Here's how the part is built. I have some questions about the finished solid (model axes, mm). Face numbers are marked on the shaded views. A direction names the side the tool comes from. Round coordinates to 2 decimals unless told otherwise and drop trailing zeros. Loops run counter-clockwise (first coordinate to the right, second up) from the corner with the lowest first, then second, coordinate; pieces in that order, holes last. Notation, with made-up numbers: (70.5, -0.75) - (95.5, -0.75) arc R32 cw to (95.5, 35.25) - close; hole circle Ø8 at (3.25, 58.25). An arc over 180 degrees is marked (long way). Answer as a JSON object with one key per item and string values. Group by question number.
1) If we mould it in two halves opening along Y, with no side actions, what happens to the marked faces 4, 5 and 6? For each: pulls with the +Y half, pulls with the -Y half, needs draft (parallel to the pull), parting line crosses it, or undercut.
2) I want a section at B-B, the plane y = -7.5. Please give me the cut outline in (x, z) (3 decimals), then the cut area to 3 significant figures.
3) If I drill on line 1 along Y through (x, z) = (19.05, 30.75); line 2 along Z through (x, y) = (17.5, 28); line 3 along Y through (x, z) = (23, 17.5), over which ranges is the centre line in solid material (lowest first)? Write a range as [from, to].
4) I want a section at D-D, the plane z = 21. Please give me the cut outline in (x, y), then the cut area to 3 significant figures.
5) I want a section at A-A, the plane x = 19.05. Please give me the cut outline in (y, z) (3 decimals), then the cut area to 3 significant figures.
6) Which directions (+Z, -Z, +X, -X, +Y, -Y) give clear straight access to the entire face, cutting with the end or side of a thin tool? Please do the marked faces 1, 2 and 3.
7) Will these pins go through, and if not, where does the flat tip stop? P1, Ø4, axis at x = 19.5, z = 20.5, coming from the +Y side; P2, Ø14, axis at x = 19.5, z = 20, coming from the -Y side; P3, Ø8, axis at y = 18, z = 29.5, coming from the +X side; P4, Ø10, axis at y = 15, z = 11.5, coming from the -X side.
8) I want a section at C-C, the plane x = 35.5. Please give me the cut outline in (y, z), then the cut area to 3 significant figures.
from build123d import *

# Parameters (mm, degrees)
F1_DEPTH = 38.1
F2_R     = 12.7
F2_R_2   = 6.35
F3_DEPTH = 15.875


with BuildPart() as f1:
    # F0 (on Right) → F1 (new body)
    with BuildSketch(Plane.YZ):
        Polygon((-31.75, 0), (0, 0), (0, 25.4), (-19.05, 25.4), (-19.05, 12.7), (-31.75, 12.7), align=None)
        Polygon((0, 25.4), (0, 0), (31.75, 0), (31.75, 12.7), (19.05, 12.7), (19.05, 25.4), align=None)
    extrude(amount=F1_DEPTH)

    # F2 (on face) → F3 (join)
    with BuildSketch(Plane.XY.offset(25.4)):
        with Locations((19.05, 0)):
            Circle(F2_R)
        with Locations((19.05, 0)):
            Circle(F2_R_2, mode=Mode.SUBTRACT)
    extrude(amount=F3_DEPTH)


solid = f1.part
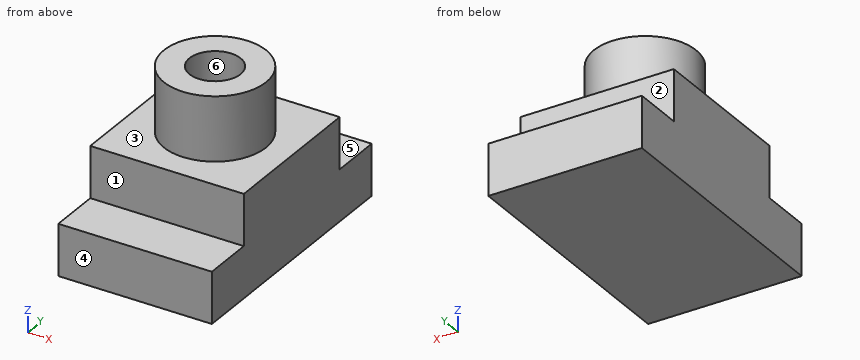
Outcome:
{
 "1": {"face 4": "pulls with the -Y half", "face 5": "needs draft", "face 6": "undercut"},
 "2": {"outline": "(0, 0) - (38.1, 0) - (38.1, 25.4) - (29.299, 25.4) - (29.299, 41.275) - (8.801, 41.275) - (8.801, 25.4) - (0, 25.4) - close", "area": "1,290 mm^2"},
 "3": {"line 1": "[-12.7, -6.35], [6.35, 12.7]", "line 2": "[0, 12.7]", "line 3": "[-19.05, 19.05]"},
 "4": {"outline": "(0, -19.05) - (38.1, -19.05) - (38.1, 19.05) - (0, 19.05) - close", "area": "1,450 mm^2"},
 "5": {"outline": "(-31.75, 0) - (31.75, 0) - (31.75, 12.7) - (19.05, 12.7) - (19.05, 25.4) - (12.7, 25.4) - (12.7, 41.275) - (6.35, 41.275) - (6.35, 25.4) - (-6.35, 25.4) - (-6.35, 41.275) - (-12.7, 41.275) - (-12.7, 25.4) - (-19.05, 25.4) - (-19.05, 12.7) - (-31.75, 12.7) - close", "area": "1,490 mm^2"},
 "6": {"face 1": "+Z, +X, -X, -Y", "face 2": "+Z, +X, -X, +Y", "face 3": "+Z"},
 "7": {"P1": "y = 19.05", "P2": "y = -19.05", "P3": "through", "P4": "x = 0"},
 "8": {"outline": "(-31.75, 0) - (31.75, 0) - (31.75, 12.7) - (19.05, 12.7) - (19.05, 25.4) - (-19.05, 25.4) - (-19.05, 12.7) - (-31.75, 12.7) - close", "area": "1,290 mm^2"}
}
